Autodesk Inventor part; units mm, degrees
ref_plane "YZ Plane" through (0, 0, 0) normal (1, 0, 0) x (0, 1, 0)
ref_plane "XZ Plane" through (0, 0, 0) normal (0, 1, 0) x (-1, 0, 0)
ref_plane "XY Plane" through (0, 0, 0) normal (0, 0, 1) x (1, 0, 0)
sketch "Sketch1" plane through (0, 0, 0) normal (0, 0, 1) x (1, 0, 0)
  line L0 (41, -16.75) -> (11.1915, -16.75)
  line L1 (41, -16.75) -> (41, -12.75)
  line L2 (-41, -12.75) -> (41, -12.75)
  line L3 (-41, -16.75) -> (-41, -12.75)
  line L4 (-11.1915, -16.75) -> (-41, -16.75)
  spline S0 degree 3 poles (-11.1915, -16.75) (-10.0304, -16.75) (-8.6395, -16.8333) (-6.313, -17.0219) (-5.0294, -17.1518) (-2.4598, -17.3597) (-1.173, -17.4271) (1.173, -17.4271) (2.4598, -17.3597) (5.0294, -17.1518) (6.313, -17.0219) (8.6395, -16.8333) (10.0304, -16.75) (11.1915, -16.75) knots 2.352794 2.352794 2.352794 2.352794 2.701135 2.701135 3.053026 3.053026 3.404917 3.404917 3.756807 3.756807 4.108698 4.108698 4.45704 4.45704 4.45704 4.45704
  line L5 (-38, -6.75) -> (-38, 6.75)
  line L6 (-38, 6.75) -> (-36, 6.75)
  line L7 (-36, 6.75) -> (-36, 12.75)
  line L8 (-41, 12.75) -> (-36, 12.75)
  line L9 (-41, -12.75) -> (-41, 12.75)
  line L10 (-41, -12.75) -> (41, -12.75)
  line L11 (41, -12.75) -> (41, 12.75)
  line L12 (36, 12.75) -> (41, 12.75)
  line L13 (36, 6.75) -> (36, 12.75)
  line L14 (36, 6.75) -> (38, 6.75)
  line L15 (38, 6.75) -> (38, -6.75)
  line L16 (38, -6.75) -> (-38, -6.75)
  line L17 (36, 12.75) -> (-36, 12.75)
  point P0 (0, 0)
extrude "Extrusion1" add sketch "Sketch1" along normal blind 3
properties part number "Cup_Dispenser_Slider_Cover"
For this review, take the finished solid that the model builds, in its own axes (mm). A direction names the side the tool comes from. Give positions to 0.01 mm unless a question says otherwise; leave off trailing zeros. Order: outer loops, then holes, each group sorted by start corner. A loop starts at its lowest first (then second) coordinate and runs counter-clockwise, first axis right, second up. Notation, with made-up numbers: (0, 32) - (13, 32) arc R24 cw to (13, 52) - close; hole circle Ø7 at (-8, 16). An arc over 180 degrees is marked (long way). Answer as a JSON object with one key per item and string values. Group by question number.
Item 1: Machinability: for faces 1 (the flat face through (26, -16.75, 1)), 2 (the flat face through (-26, -16.75, 1)), which of the approach directions +Z, -Z, +X, -X, +Y, -Y give a long, thin tool a straight path to every point of the face, cutting with its end or side? Answer none if there is none.
Item 2: Wall thickness on line 1 along Y through (x, z) = (0.5, 0.3); line 2 along Y through (x, z) = (-24, 0.25): over which ranges is each line inside the solid? List them lowest first.
Item 3: Clearance check with flat-ended pins moving along their axes: pin 1 Ø8 at (x, y) = (-6, 2.5) entering from -Z; pin 2 Ø1.5 at (x, z) = (23, 1) entering from -Y. State where each tip first meets the part, or that it passes through.
Item 4: Take a section at A-A on x = 21.5. Give the boundary of the cut face in (y, z).
Reported:
{
 "1": {"face 1": "+Z, -Z, +X, -Y", "face 2": "+Z, -Z, -X, -Y"},
 "2": {"line 1": "-17.42 to 12.75", "line 2": "-16.75 to 12.75"},
 "3": {"pin 1": "z = 0", "pin 2": "y = -16.75"},
 "4": {"outline": "(-16.75, 0) - (12.75, 0) - (12.75, 3) - (-16.75, 3) - close"}
}
